Autodesk Inventor part; units mm, degrees
ref_plane "YZ Plane" through (0, 0, 0) normal (1, 0, 0) x (0, 1, 0)
ref_plane "XZ Plane" through (0, 0, 0) normal (0, 1, 0) x (-1, 0, 0)
ref_plane "XY Plane" through (0, 0, 0) normal (0, 0, 1) x (1, 0, 0)
sketch "Sketch2" plane through (0, 0, 0) normal (0, 1, 0) x (-1, 0, 0)
  line L0 (10.6557, -7.541) -> (-9.3443, -7.541)
  line L1 (-9.3443, -7.541) -> (-9.3443, 12.459)
  line L2 (-9.3443, 12.459) -> (10.6557, 12.459)
  line L3 (10.6557, 12.459) -> (10.6557, -7.541)
  point P0 (0, 0)
  dimension "d10" = 20
  dimension "d11" = 20
extrude "Extrusion3" add sketch "Sketch2" along normal blind 8
sketch "Sketch3" plane through (0, 8, 0) normal (0, 1, 0) x (1, 0, 0)
  line L0 (9.3443, 7.541) -> (-10.6557, 7.541)
  line L1 (-10.6557, 7.541) -> (-10.6557, -12.459)
  line L2 (-10.6557, -12.459) -> (9.3443, -12.459)
  line L3 (9.3443, -12.459) -> (9.3443, 7.541)
  line L4 (-9.6557, -11.459) -> (-9.6557, 6.541)
  line L5 (-9.6557, 6.541) -> (8.3443, 6.541)
  line L6 (8.3443, 6.541) -> (8.3443, -11.459)
  line L7 (8.3443, -11.459) -> (4.3443, -11.459)
  line L8 (4.3443, -11.459) -> (4.3443, 2.541)
  line L9 (4.3443, 2.541) -> (-5.6557, 2.541)
  line L10 (-5.6557, 2.541) -> (-5.6557, -11.459)
  line L11 (-5.6557, -11.459) -> (-9.6557, -11.459)
  line L12 (-9.6557, 6.541) -> (-10.6557, 6.541) construction
  line L13 (8.3443, 6.541) -> (9.3443, 6.541) construction
  line L14 (-9.6557, 6.541) -> (-9.6557, 7.541) construction
  point P0 (0, 0)
  dimension "d14" = 10
  dimension "d15" = 4
  dimension "d16" = 4
  dimension "d17" = 1
  dimension "d18" = 14
extrude "Extrusion4" add sketch "Sketch3" along normal blind 20 contours L4 L5 L6 L7 L8 L9 L10 L11
sketch "Sketch4" plane through (8.3443, 8, -6.541) normal (0, 0, -1) x (-1, 0, 0)
  circle A0 centre (9, 9.875) radius 2.125
  line L0 (9, 9.875) -> (0, 9.875) construction
  line L1 (0, 0) -> (0, 20)
  line L2 (9, 9.875) -> (18, 9.875) construction
  line L3 (18, 0) -> (18, 20)
  line L4 (0, 20) -> (18, 20)
  point P0 (8.3443, -8)
  dimension "d21" = 4.25
  dimension "d22" = 8
extrude "Extrusion5" cut sketch "Sketch4" against normal up to next
properties part number "XPulleySupport"
Build history of the part. All positions in model axes, mm. A direction names the side the tool comes from. Coordinates: 2 decimals unless noted, no trailing zeros. Order: outer loops, then holes, each group sorted by start corner. A loop starts at its lowest first (then second) coordinate and runs counter-clockwise, first axis right, second up. Notation, with made-up numbers: M -19.5,80.25 L 7.5,80.25 A20 ccw 7.5,100.25 Z; hole C 83.25,-4 d9. An arc over 180 degrees is marked long. One line per question, with ' | ' between items. Start each with the question number.
1. Cut at C-C (x = 7.75). Write the cut outline in (y, z).
2. Wall check: line 1 along X through (y, z) = (16.5, 5.25); line 2 along Z through (x, y) = (-6.75, 21); line 3 along Y through (x, z) = (0.5, 5.75). Give the ranges that are in metal, low to high. Write a range as [from, to].
3. Cut at A-A (x = -2.25). Write the cut outline in (y, z), plus the area to 3 significant figures.
4. Cut at D-D (z = 5.5). Write the cut outline in (x, y), plus the area to 3 significant figures.
5. Mould opens along X. For faces 1 (the face through (-9.656, 18, 3)), 2 (the face through (4.344, 18, 5)), 3 (the face through (-1, 28, -4)) say: +X half, -X half, draft (parallel to the pull), parting line (faces both ways), or undercut.
6. Flat gauge pins, fed straight in: P1, Ø1.5, axis at x = -4.5, z = 3.5, coming from the +Y side; P2, Ø10, axis at y = 23, z = 1, coming from the +X side; P3, Ø7, axis at x = -0.66, y = 17.88, coming from the -Z side. Where does each tip first touch, or does it go through?
7. Tool access for faces 4 (the face through (-5.656, 18, 4)), 5 (the face through (-8, 18, 11.459)), 6 (the face through (8.344, 18, 2)): list every direction of +Z, -Z, +X, -X, +Y, -Y with a clear straight run to the whole face (end or side of a thin tool).
8. Cut at B-B (y = 12.75). Write the cut outline in (x, z), plus the area to 3 significant figures.
The answers:
1) outline: M 0,-7.54 L 8,-7.54 L 8,-6.54 L 28,-6.54 L 28,11.46 L 8,11.46 L 8,12.46 L 0,12.46 Z
2) line 1: x = [-9.66, -5.66], [4.34, 8.34] | line 2: z = [-6.54, 11.46] | line 3: y = [0, 8]
3) outline: M 0,-7.54 L 8,-7.54 L 8,-6.54 L 16.47,-6.54 L 16.47,-2.54 L 8,-2.54 L 8,12.46 L 0,12.46 Z; M 19.28,-6.54 L 28,-6.54 L 28,-2.54 L 19.28,-2.54 Z | area: 229 mm2
4) outline: M -10.66,0 L 9.34,0 L 9.34,8 L 8.34,8 L 8.34,28 L 4.34,28 L 4.34,8 L -5.66,8 L -5.66,28 L -9.66,28 L -9.66,8 L -10.66,8 Z | area: 320 mm2
5) face 1: -X half | face 2: undercut | face 3: draft
6) P1: stops at y = 8 | P2: stops at x = 8.34 | P3: stops at z = -6.54
7) face 4: +Z, +Y | face 5: +Z, +X, -X, +Y | face 6: +Z, -Z, +X, +Y
8) outline: M -9.66,-6.54 L 8.34,-6.54 L 8.34,11.46 L 4.34,11.46 L 4.34,-2.54 L -5.66,-2.54 L -5.66,11.46 L -9.66,11.46 Z | area: 184 mm2
